Verification items for the finished model (mm, model axes). Give positions to 0.01 mm unless a question says otherwise; leave off trailing zeros. Write each loop counter-clockwise with the first axis right and the second up, starting at its lowest first coordinate (ties: lowest second). Pieces come first, ordered by that corner, then holes. Notation, with made-up numbers: (28.5, 81.5) - (41.5, 81.5) arc R22 cw to (41.5, 100.5) - close; hole circle Ø9 at (-11, 12.5). An arc over 180 degrees is marked (long way). Put each result on its own line as item: value.
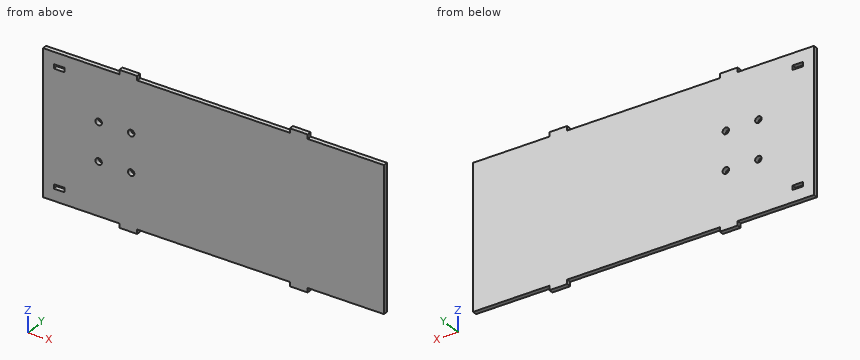
from build123d import *

# Parameters (mm, degrees)
MAIN_FRAME_DEPTH   = 3.175
SKETCH2_R          = 2.276969522
FRONT_WHEEL_DEPTH  = 4.175
SKETCH4_W          = 7.62
SKETCH4_H          = 3.048
SENSOR_HOLES_DEPTH = 4.175


with BuildPart() as part:
    # Sketch1 → Main Frame (new body)
    with BuildSketch(Plane(origin=(0, 0, 0), x_dir=(1, 0, 0), z_dir=(0, 1, 0))):
        Polygon((0, 0), (41.275, 0), (41.275, -3.048), (53.975, -3.048), (53.975, 0), (161.925, 0), (161.925, -3.048), (174.625, -3.048), (174.625, 0), (228.6, 0), (228.6, 101.6), (174.625, 101.6), (174.625, 104.648), (161.925, 104.648), (161.925, 101.6), (53.975, 101.6), (53.975, 104.648), (41.275, 104.648), (41.275, 101.6), (0, 101.6), (-12.7, 101.6), (-12.7, 0), align=None)
    extrude(amount=MAIN_FRAME_DEPTH)

    # Sketch2 → Front Wheel (cut, through all)
    with BuildSketch(Plane(origin=(0, 3.175, 0), x_dir=(1, 0, 0), z_dir=(0, 1, 0))):
        with Locations((26.67, 64.29375)):
            Circle(SKETCH2_R)
        with Locations((49.68875, 64.29375)):
            Circle(SKETCH2_R)
        with Locations((49.68875, 37.30625)):
            Circle(SKETCH2_R)
        with Locations((26.67, 37.30625)):
            Circle(SKETCH2_R)
    extrude(amount=-FRONT_WHEEL_DEPTH, mode=Mode.SUBTRACT)

    # Sketch4 → Sensor Holes (cut, through all)
    with BuildSketch(Plane(origin=(0, 3.175, 0), x_dir=(1, 0, 0), z_dir=(0, 1, 0))):
        with Locations((-1.27, 91.707882035)):
            Rectangle(SKETCH4_W, SKETCH4_H)
        with Locations((-1.27, 9.892117965)):
            Rectangle(SKETCH4_W, SKETCH4_H)
    extrude(amount=-SENSOR_HOLES_DEPTH, mode=Mode.SUBTRACT)


solid = part.part
Q1. Section check A-A, the plane x = 26.67. Record the cut outline in (y, z) (3 decimals), plus the area to 3 significant figures.
Answers follow:
outline: (0, -101.6) - (3.175, -101.6) - (3.175, -66.571) - (0, -66.571) - close; (0, -62.017) - (3.175, -62.017) - (3.175, -39.583) - (0, -39.583) - close; (0, -35.029) - (3.175, -35.029) - (3.175, 0) - (0, 0) - close
area: 294 mm2
Q2. Section check B-B, the plane y = 1.5. Give the number of separate pieces and of enclosed holes in the cut face, plus the area to 3 significant figures.
Answers follow:
separate pieces: 1
enclosed holes: 6
area: 24,600 mm2
Q3. Section check C-C, the plane x = 126.5. Record the cut outline in (y, z) (3 decimals).
Answers follow:
outline: (0, -101.6) - (3.175, -101.6) - (3.175, 0) - (0, 0) - close
Q4. Scan lines: line 1 along Z through (x, y) = (26.67, 2.35); line 2 along Z through (x, y) = (36.5, 2.8). Record each from-to range of solid material in increasing order.
Answers follow:
line 1: z = -101.6 to -66.57, -62.02 to -39.58, -35.03 to 0
line 2: z = -101.6 to 0
Q5. Go/stop test with flat-tipped pins: pin 1 Ø1.5 at (y, z) = (1.5, 1) entering from -X (3 decimals); pin 2 Ø1.6 at (x, y) = (83, 1.5) entering from +Z. Record where each tip stops, or that it passes through.
Answers follow:
pin 1: stops at x = 41.275
pin 2: stops at z = 0
